Verification items for the finished model (mm, model axes). A direction names the side the tool comes from. Round coordinates to 2 decimals unless told otherwise and drop trailing zeros. Loops run counter-clockwise (first coordinate to the right, second up) from the corner with the lowest first, then second, coordinate; pieces in that order, holes last. Notation, with made-up numbers: (36, -1.75) -> (80, -1.75) arc R31 ccw to (80, 28.25) -> close; hole circle Ø6 at (77.5, 45.25). An arc over 180 degrees is marked (long way). Write item = value, one per line.
```python
from build123d import *

# Parameters (mm, degrees)
SKETCH1_R           = 1.1
BOSS_EXTRUDE1_DEPTH = 4.5
SKETCH2_R           = 3
CUT_EXTRUDE2_DEPTH  = 10
CUT_EXTRUDE4_START  = -6
CUT_EXTRUDE4_DEPTH  = 17
CUT_EXTRUDE6_DEPTH  = 23
FILLET4_R           = 3
FILLET1_R           = 0.5
SKETCH5_R           = 1.75
CUT_EXTRUDE5_DEPTH  = 1


with BuildPart() as part:
    # Sketch1 → Boss-Extrude1 (new body)
    with BuildSketch(Plane.XY):
        with BuildLine():
            Line((-15, 7), (0, 7))
            ThreePointArc((0, 7), (7, 0), (0, -7))
            Line((0, -7), (-15, -7))
            Line((-15, -7), (-15, 7))
        make_face()
        with Locations((-12, 3.5)):
            Circle(SKETCH1_R, mode=Mode.SUBTRACT)
        with Locations((-12, -3.5)):
            Circle(SKETCH1_R, mode=Mode.SUBTRACT)
    extrude(amount=BOSS_EXTRUDE1_DEPTH)

    # Sketch2 → Cut-Extrude2 (cut)
    with BuildSketch(Plane(origin=(0, 0, 0), x_dir=(-1, 0, 0), z_dir=(0, 0, -1))):
        Circle(SKETCH2_R)
    extrude(amount=-CUT_EXTRUDE2_DEPTH, mode=Mode.SUBTRACT)

    # Sketch7 → Cut-Extrude4 (cut, through all)
    with BuildSketch(Plane.ZY.offset(15).offset(CUT_EXTRUDE4_START)):
        Polygon((2.8, 5.55), (0.6, 5.55), (0.6, 0), (4.5, 0), (4.5, 4.95), (3.4, 4.95), align=None)
        Polygon((4.5, 0), (0.6, 0), (0.6, -5.55), (2.8, -5.55), (3.4, -4.95), (4.5, -4.95), align=None)
    extrude(amount=-CUT_EXTRUDE4_DEPTH, mode=Mode.SUBTRACT)

    # Sketch8 → Cut-Extrude6 (cut, through all)
    with BuildSketch(Plane.ZY.offset(15)):
        with BuildLine():
            Line((3.2, 1.363340016), (3.2, -1.363340016))
            ThreePointArc((3.2, -1.363340016), (3.404046985, -1.855953015), (3.896659984, -2.06))
            Line((3.896659984, -2.06), (4.5, -2.06))
            Line((4.5, -2.06), (4.5, 2.06))
            Line((4.5, 2.06), (3.896659984, 2.06))
            ThreePointArc((3.896659984, 2.06), (3.404046985, 1.855953015), (3.2, 1.363340016))
        make_face()
    extrude(amount=-CUT_EXTRUDE6_DEPTH, mode=Mode.SUBTRACT)

    # Fillet4
    fillet4_edges = [part.edges().sort_by_distance(p)[0] for p in [
        (-15, -7, 2.25),
        (-15, 7, 2.25),
    ]]
    fillet(fillet4_edges, radius=FILLET4_R)

    # Fillet1
    fillet1_edges = [part.edges().sort_by_distance(p)[0] for p in [
        (-6, 7, 0),
        (7, 0, 0),
        (-15, 0, 0),
        (-6, -7, 0),
        (-14.121320344, -6.121320344, 0),
        (-14.121320344, 6.121320344, 0),
    ]]
    fillet(fillet1_edges, radius=FILLET1_R)

    # Sketch5 → Cut-Extrude5 (cut)
    with BuildSketch(Plane.XY):
        with Locations((-12, 3.5)):
            Circle(SKETCH5_R)
        with Locations((-12, -3.5)):
            Circle(SKETCH5_R)
    extrude(amount=CUT_EXTRUDE5_DEPTH, mode=Mode.SUBTRACT)


solid = part.part
```
(1) Sectioned sample at B-B, the plane z = 1.9. Record the cut outline in (x, y), and give its area (3 significant figures).
Filled sheet:
outline = (-15, -4) arc R3 ccw to (-12, -7) -> (0, -7) arc R7 ccw to (4.27, -5.55) -> (-9, -5.55) -> (-9, 5.55) -> (4.27, 5.55) arc R7 ccw to (0, 7) -> (-12, 7) arc R3 ccw to (-15, 4) -> close; hole circle Ø2.2 at (-12, -3.5); hole circle Ø2.2 at (-12, 3.5)
area = 107 mm2
(2) Set-up check for faces 1 (the face through (-2, -5.55, 2)), 2 (the face through (-12, -5, 1)), 3 (the face through (-14.1, 6.14, 2.53)), 4 (the face through (-2, -4.95, 4)), 5 (the face through (-12, 0, 3.2)): record each of +Z, -Z, +X, -X, +Y, -Y from which the full face is reachable in a straight line by a thin tool's end or side.
Filled sheet:
face_1 = +X
face_2 = -Z
face_3 = +Z, -Z, -X, +Y
face_4 = +Z, +X
face_5 = +Z, +X, -X
(3) Sectioned sample at C-C, the plane x = -11.25. Record the cut outline in (y, z), and give its area (3 significant figures).
Filled sheet:
outline = (-7, 0.5) arc R0.5 ccw to (-6.5, 0) -> (-5.08, 0) -> (-5.08, 1) -> (-4.3, 1) -> (-4.3, 4.5) -> (-7, 4.5) -> close; (-2.7, 1) -> (-1.92, 1) -> (-1.92, 0) -> (1.92, 0) -> (1.92, 1) -> (2.7, 1) -> (2.7, 4.5) -> (2.06, 4.5) -> (2.06, 3.9) arc R0.7 cw to (1.36, 3.2) -> (-1.36, 3.2) arc R0.7 cw to (-2.06, 3.9) -> (-2.06, 4.5) -> (-2.7, 4.5) -> close; (4.3, 1) -> (5.08, 1) -> (5.08, 0) -> (6.5, 0) arc R0.5 ccw to (7, 0.5) -> (7, 4.5) -> (4.3, 4.5) -> close
area = 40.2 mm2
(4) Draft check along Y on faces 6 (the face through (-2, 4.95, 4)), 7 (the face through (-14.14, -6.1, 2.53)), 8 (the face through (-15, 0, 2)). Enter one of: released by +Y, released by -Y, zero draft, split by the parting line, or undercut.
Filled sheet:
face_6 = undercut
face_7 = released by -Y
face_8 = zero draft
(5) Go/stop test with flat-tipped pins: pin 1 Ø3 at (x, y) = (-12, -3.5) entering from +Z; pin 2 Ø2 at (y, z) = (0, 3.5) entering from +X; pin 3 Ø5.5 at (x, y) = (-1, 2) entering from +Z; pin 4 Ø0.5 at (x, z) = (-12.5, 4) entering from -Y. Record where each tip stops, or that it passes through.
Filled sheet:
pin_1 = 4.5
pin_2 = -9
pin_3 = 0.6
pin_4 = -6.99
(6) Sectioned sample at A-A, the plane x = -4. Record the cut outline in (y, z), and give its area (3 significant figures).
Filled sheet:
outline = (-7, 0.5) arc R0.5 ccw to (-6.5, 0) -> (6.5, 0) arc R0.5 ccw to (7, 0.5) -> (7, 4.5) -> (4.95, 4.5) -> (4.95, 3.4) -> (5.55, 2.8) -> (5.55, 0.6) -> (-5.55, 0.6) -> (-5.55, 2.8) -> (-4.95, 3.4) -> (-4.95, 4.5) -> (-7, 4.5) -> close
area = 21.3 mm2
(7) Material ranges on probe 1 along Y at (x, z) = (-12, 0.55); probe 2 along Y at (x, z) = (-12, 3.6); probe 3 along Y at (x, z) = (-6.5, 0.45), recorded low to high. Write a range as from..to.
Filled sheet:
probe_1 = -7..-5.25, -1.75..1.75, 5.25..7
probe_2 = -7..-4.6, -2.4..-1.99, 1.99..2.4, 4.6..7
probe_3 = -7..7
